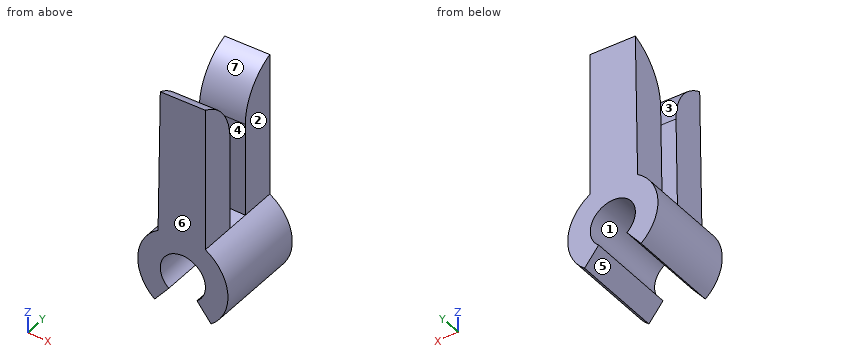
from build123d import *

# Parameters (mm, degrees)
F1_DEPTH    = 6.35
F2_W        = 1.524
F2_H        = 10.16
F3_DEPTH    = 25.4
F4_T1_DEPTH = 20.8982128859
F5_T1_DEPTH = 20.8982128859


# Not quite as in the source:
# - a fillet or chamfer that OpenCascade refuses, or shapes differently, is made with other operations: its cross-section is extruded or revolved along the edge and cut away or added


with BuildPart() as f1:
    # F0 (on Front) → F1 (new body)
    with BuildSketch(Plane.XZ):
        with BuildLine():
            Line((0.9929372138, -1.2386411666), (1.9858744275, -2.4772823331))
            ThreePointArc((1.9858744275, -2.4772823331), (3.1658183857, 0.2412860305), (1.5875, 2.749630657))
            Line((1.5875, 2.749630657), (1.5875, 12.909630657))
            Line((1.5875, 12.909630657), (-1.58600151, 12.8120951952))
            Line((-1.58600151, 12.8120951952), (-1.7437092207, 2.653319271))
            ThreePointArc((-1.7437092207, 2.653319271), (-3.1714691788, 0.1496938466), (-1.9858744275, -2.4772823331))
            Line((-1.9858744275, -2.4772823331), (-0.9929372138, -1.2386411666))
            ThreePointArc((-0.9929372138, -1.2386411666), (0, 1.5875), (0.9929372138, -1.2386411666))
        make_face()
    extrude(amount=F1_DEPTH)

    # F2 (on face) → F3 (cut)
    with BuildSketch(Plane.YZ.offset(1.5875)):
        with Locations((-3.175, 7.829630657)):
            Rectangle(F2_W, F2_H)
    extrude(amount=-F3_DEPTH, mode=Mode.SUBTRACT)

    # F4: fillet of radius 3.81 on 1 edges, made by hand

    # F4_s2 → F4_t1 (cut)
    with BuildSketch(Plane(origin=(10.839820428, 0, 0.3331546837), x_dir=(0, 1, 0), z_dir=(-0.9995280346, 0, -0.0307198305))):
        with BuildLine():
            ThreePointArc((-6.35, -12.8547700275), (-4.597502421, -11.4541342134), (-3.937, -9.3101274503))
            Line((-3.937, -9.3101274503), (-3.937, -12.8547700275))
            Line((-3.937, -12.8547700275), (-6.35, -12.8547700275))
        make_face()
    extrude(amount=F4_T1_DEPTH, mode=Mode.SUBTRACT)

    # F5: fillet of radius 3.81 on 1 edges, made by hand

    # F5_s2 → F5_t1 (cut)
    with BuildSketch(Plane(origin=(-10.0485292251, 0, -0.308834874), x_dir=(0, 1, 0), z_dir=(0.9995280346, 0, 0.0307198305))):
        with BuildLine():
            ThreePointArc((0, 12.8547700275), (-1.752497579, 11.4541342134), (-2.413, 9.3101274503))
            Line((-2.413, 9.3101274503), (-2.413, 12.8547700275))
            Line((-2.413, 12.8547700275), (0, 12.8547700275))
        make_face()
    extrude(amount=F5_T1_DEPTH, mode=Mode.SUBTRACT)


solid = f1.part
Here's how the part is built. I have some questions about the finished solid (model axes, mm). Face numbers are marked on the shaded views. A direction names the side the tool comes from. Give positions to 0.01 mm unless a question says otherwise; leave off trailing zeros. Order: outer loops, then holes, each group sorted by start corner. A loop starts at its lowest first (then second) coordinate and runs counter-clockwise, first axis right, second up. Notation, with made-up numbers: (39, 54.5) -> (96, 54.5) arc R30 ccw to (96, 87.5) -> close; hole circle Ø2 at (-35, 68.25). An arc over 180 degrees is marked (long way). Use a Markdown table: item, result. Add a question column.
Item 1: Will these pins go through, and if not, where does the flat tip stop? pin 1 (1.9 mm diameter, centred on y = -5.5, z = 9.5, fed in from +X); pin 2 (0.8 mm diameter, centred on x = -0.5, y = -3, fed in from +Z); pin 3 (1.5 mm diameter, centred on x = 2.5, y = -2, fed in from +Z).
Item 2: Imagine slicing it at C-C on z = 7.25. Please give me the cut outline in (x, y), plus the area to 3 significant figures.
Item 3: For the marked faces 1, 2, 3 and 4, which set-ups out of +Z, -Z, +X, -X, +Y, -Y let a thin tool reach every point of the face, with its end or its side?
Item 4: I need wall thicknesses on line 1 (Y direction, x = -0.75, z = 6); line 2 (X direction, y = -2, z = 0) (1 decimal); line 3 (Z direction, x = 1.25, y = -1.75). Which ranges of each line are inside material? Lowest first, please.
Item 5: If we mould it in two halves opening along Y, with no side actions, what happens to the marked faces 5, 6 and 7? For each: pulls with the +Y half, pulls with the -Y half, needs draft (parallel to the pull), parting line crosses it, or undercut.
Item 6: Imagine slicing it at D-D on x = -2.25. Please give me the cut outline in (y, z).
Data:
| question | item | result |
|---|---|---|
| 1 | pin 1 | stops at x = 1.59 |
| 1 | pin 2 | stops at z = 2.75 |
| 1 | pin 3 | stops at z = 2.65 |
| 2 | outline | (-1.67, -6.35) -> (1.59, -6.35) -> (1.59, -3.94) -> (-1.67, -3.94) -> close; (-1.67, -2.41) -> (1.59, -2.41) -> (1.59, 0) -> (-1.67, 0) -> close |
| 2 | area | 15.7 mm² |
| 3 | face 1 | +Y, -Y |
| 3 | face 2 | +Z, +X, +Y, -Y |
| 3 | face 3 | +Z, -X |
| 3 | face 4 | +Z, +X, -X |
| 4 | line 1 | y = -6.35 to -3.94, -2.41 to 0 |
| 4 | line 2 | x = -3.2 to -1.6, 1.6 to 3.2 |
| 4 | line 3 | z = -1.56 to -0.98, 0.98 to 11.5 |
| 5 | face 5 | needs draft |
| 5 | face 6 | pulls with the -Y half |
| 5 | face 7 | undercut |
| 6 | outline | (-6.35, -2.24) -> (0, -2.24) -> (0, 2.24) -> (-6.35, 2.24) -> close |
